Could you check a few things on this drawing? It's one solid part, dimensions in mm from its lowest x, y, z. Coordinates: 2 decimals unless noted, no trailing zeros. Write each loop counter-clockwise with the first axis right and the second up, starting at its lowest first coordinate (ties: lowest second). Pieces come first, ordered by that corner, then holes. Notation, with made-up numbers: (8, 51.25) - (42, 51.25) arc R26 ccw to (42, 76.25) - close; hole circle Ø11 at (-36, 40.25). An arc over 180 degrees is marked (long way). Answer as a JSON object with one key per item and string values. Group by question number.
1) We'd pull the mould along Y, two halves only. Please class the marked faces 1, 2 and 3: released by +Y, released by -Y, zero draft, split by the parting line, or undercut.
2) If we section it at A-A (y = 6): Write out the boundary of the cut face in (x, z), plus the area to 3 significant figures.
3) If we section it at C-C (z = 1.45): Write out the boundary of the cut face in (x, y), plus the area to 3 significant figures.
4) Please list where these lines run through material, in increasing order: line 1 along Y through (x, z) = (6, 1); line 2 along X through (y, z) = (5.75, 1.25); line 3 along Y through (x, z) = (7, 0.8).
5) Will these pins go through, and if not, where does the flat tip stop? pin 1 Ø3 at (x, y) = (7.5, 4.5) entering from +Z; pin 2 Ø1 at (y, z) = (8, 1) entering from -X.
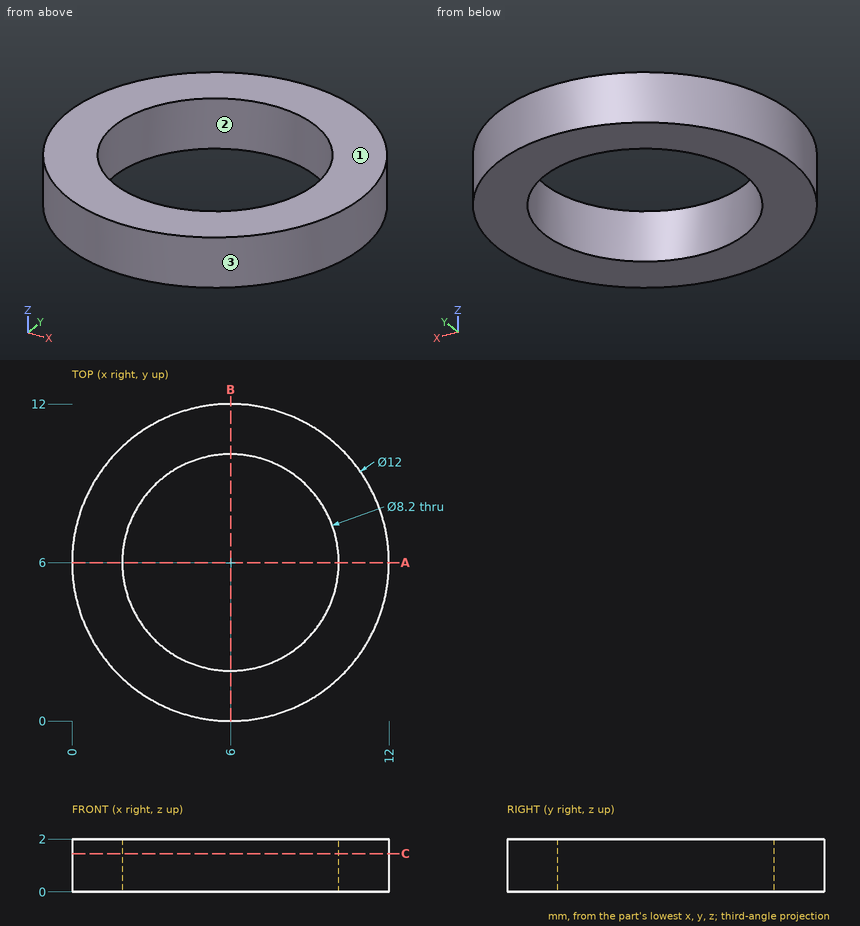
Here are the results:
{
 "1": {"face 1": "zero draft", "face 2": "undercut", "face 3": "split by the parting line"},
 "2": {"outline": "(0, 0) - (1.9, 0) - (1.9, 2) - (0, 2) - close; (10.1, 0) - (12, 0) - (12, 2) - (10.1, 2) - close", "area": "7.60 mm²"},
 "3": {"outline": "circle Ø12 at (6, 6); hole circle Ø8.2 at (6, 6)", "area": "60.3 mm²"},
 "4": {"line 1": "y = 0 to 1.9, 10.1 to 12", "line 2": "x = 0.01 to 1.91, 10.09 to 11.99", "line 3": "y = 0.08 to 2.02, 9.98 to 11.92"},
 "5": {"pin 1": "passes through", "pin 2": "stops at x = 0.19"}
}
